```python
from build123d import *

# Parameters (mm, degrees)
SKETCH1_W           = 127
SKETCH1_H           = 152.4
BOSS_EXTRUDE2_DEPTH = 1612.9
SKETCH2_R           = 19.05
CUT_EXTRUDE1_DEPTH  = 152.4
SKETCH3_R           = 19.05
CUT_EXTRUDE2_DEPTH  = 152.4


with BuildPart() as part:
    # Sketch1 → Boss-Extrude2 (new body)
    with BuildSketch(Plane(origin=(0, 0, 0), x_dir=(1, 0, 0), z_dir=(0, 1, 0))):
        with Locations((63.5, 76.2)):
            Rectangle(SKETCH1_W, SKETCH1_H)
    extrude(amount=BOSS_EXTRUDE2_DEPTH)

    # Sketch2 → Cut-Extrude1 (cut)
    with BuildSketch(Plane(origin=(127, 0, 0), x_dir=(0, 0, -1), z_dir=(1, 0, 0))):
        with Locations((25.4, 25.4)):
            Circle(SKETCH2_R)
    extrude(amount=-CUT_EXTRUDE1_DEPTH, mode=Mode.SUBTRACT)

    # Sketch3 → Cut-Extrude2 (cut)
    with BuildSketch(Plane(origin=(127, 0, 0), x_dir=(0, 0, -1), z_dir=(1, 0, 0))):
        with Locations((76.2, 1587.5)):
            Circle(SKETCH3_R)
    extrude(amount=-CUT_EXTRUDE2_DEPTH, mode=Mode.SUBTRACT)


solid = part.part
```
Input: part model. Units: mm. Frame: model coordinates. Give positions to 0.01 mm unless a question says otherwise; leave off trailing zeros. Loops run counter-clockwise (first coordinate to the right, second up) from the corner with the lowest first, then second, coordinate; pieces in that order, holes last. Notation, with made-up numbers: (54.5, 28.5) -> (87.5, 28.5) arc R35 cw to (87.5, 63.5) -> close; hole circle Ø11 at (68, 31.5). An arc over 180 degrees is marked (long way). Use a Markdown table: item, result.
Q1. Section query B-B, the plane z = -25.4. Return the cut outline in (x, y), plus the area to 3 significant figures.
Entries:
| item | result |
|---|---|
| outline | (0, 0) -> (127, 0) -> (127, 6.35) -> (0, 6.35) -> close; (0, 44.45) -> (127, 44.45) -> (127, 1612.9) -> (0, 1612.9) -> close |
| area | 200,000 mm² |
Q2. Section query A-A, the plane y = 25.4. Return the cut outline in (x, z), plus the area to 3 significant figures.
Entries:
| item | result |
|---|---|
| outline | (0, -152.4) -> (127, -152.4) -> (127, -44.45) -> (0, -44.45) -> close; (0, -6.35) -> (127, -6.35) -> (127, 0) -> (0, 0) -> close |
| area | 14,500 mm² |
Q3. Ray query, probe 1 along Y at (x, z) = (53.5, -76.2); probe 2 along Y at (x, z) = (63.5, -25.4); probe 3 along Z at (x, y) = (70, 25). Return the intervals inside material, ascending. Write a range as from..to.
Entries:
| item | result |
|---|---|
| probe 1 | y = 0..1568.45, 1606.55..1612.9 |
| probe 2 | y = 0..6.35, 44.45..1612.9 |
| probe 3 | z = -152.4..-44.45, -6.35..0 |
Q4. Pull-direction query (Z, two-part tool) for faces 1 (the cylindrical face through (64.389, 6.803, -21.27)), 2 (the flat face through (63, 795, -152.4)), 3 (the flat face through (63, 795, 0)), 4 (the flat face through (63, 0, -77)); classes: pulls with the +Z half, pulls with the -Z half, needs draft (parallel to the pull), parting line crosses it, or undercut.
Entries:
| item | result |
|---|---|
| face 1 | undercut |
| face 2 | pulls with the -Z half |
| face 3 | pulls with the +Z half |
| face 4 | needs draft |
